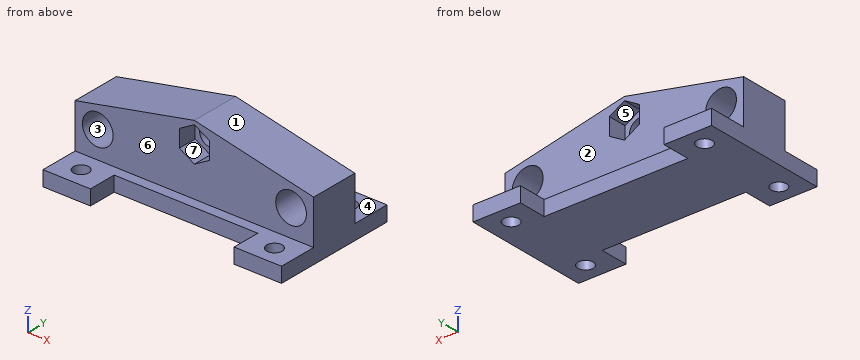
```python
from build123d import *

# Parameters (mm, degrees)
F0_W      = 100.584
F0_H      = 53.34
F1_DEPTH  = 6.35
F2_W      = 100.584
F2_H      = 20.828
F3_DEPTH  = 29.21
F5_DEPTH  = 8
F7_DEPTH  = 8
F9_D      = 9
F11_D     = 12.954
F13_D     = 6.528
F14_W     = 60.584
F14_H     = 12
F15_DEPTH = 6.35
F16_W     = 60.584
F16_H     = 12
F17_DEPTH = 6.35
F19_DEPTH = 20.828


with BuildPart() as f1:
    # F0 (on Top) → F1 (new body)
    with BuildSketch(Plane.XY):
        with Locations((2.149524, 1.085451)):
            Rectangle(F0_W, F0_H)
    extrude(amount=F1_DEPTH)

    # F2 (on face) → F3 (join)
    with BuildSketch(Plane.XY.offset(6.35)):
        with Locations((2.149524, 1.085451)):
            Rectangle(F2_W, F2_H)
    extrude(amount=F3_DEPTH)

    # F4 (on face) → F5 (cut)
    with BuildSketch(Plane.XZ.offset(9.328549)):
        Polygon((8.489524, 23.020798), (8.489524, 30.341599), (2.149524, 34.002), (-4.190476, 30.341599), (-4.190476, 23.020798), (2.149524, 19.360397), align=None)
    extrude(amount=-F5_DEPTH, mode=Mode.SUBTRACT)

    # F6 (on face) → F7 (cut)
    with BuildSketch(Plane(origin=(0, 11.499451, 0), x_dir=(-1, 0, 0), z_dir=(0, 1, 0))):
        Polygon((4.190476, 23.020798), (4.190476, 30.341599), (-2.149524, 34.002), (-8.489524, 30.341599), (-8.489524, 23.020798), (-2.149524, 19.360397), align=None)
    extrude(amount=-F7_DEPTH, mode=Mode.SUBTRACT)

    # F9 (through all)
    with Locations(Plane(origin=(0, 11.499451, 0), x_dir=(-1, 0, 0), z_dir=(0, 1, 0))):
        with Locations((-2.149524, 26.681199)):
            Hole(F9_D / 2)

    # F11 (through all)
    with Locations(Plane.XZ.offset(9.328549)):
        with Locations((42.916524, 17.656), (-38.617476, 17.656)):
            Hole(F11_D / 2)

    # F13 (through all)
    with Locations(Plane.XY.offset(6.35)):
        with Locations((-38.617476, -17.710549), (-38.617476, 19.881451), (42.916524, 19.881451), (42.916524, -17.710549)):
            Hole(F13_D / 2)

    # F14 (on face) → F15 (cut, through all)
    with BuildSketch(Plane.XY.offset(6.35)):
        with Locations((2.149524, 21.755451)):
            Rectangle(F14_W, F14_H)
    extrude(amount=-F15_DEPTH, mode=Mode.SUBTRACT)

    # F16 (on face) → F17 (cut, through all)
    with BuildSketch(Plane.XY.offset(6.35)):
        with Locations((2.149524, -19.584549)):
            Rectangle(F16_W, F16_H)
    extrude(amount=-F17_DEPTH, mode=Mode.SUBTRACT)

    # F18 (on face) → F19 (cut, through all)
    with BuildSketch(Plane.XZ.offset(9.328549)):
        Polygon((-48.142476, 25.013294), (2.149524, 35.56), (-48.142476, 35.56), align=None)
        Polygon((52.441524, 35.56), (2.149524, 35.56), (52.441524, 25.013294), align=None)
    extrude(amount=-F19_DEPTH, mode=Mode.SUBTRACT)


solid = f1.part
```
Verification items for the finished model (mm, model axes). Face numbers are marked on the shaded views. A direction names the side the tool comes from. Coordinates: 2 decimals unless noted, no trailing zeros. Order: outer loops, then holes, each group sorted by start corner. A loop starts at its lowest first (then second) coordinate and runs counter-clockwise, first axis right, second up. Notation, with made-up numbers: (-36, 62) -> (-31, 62) arc R14 cw to (-31, 80) -> close; hole circle Ø6 at (0, 76.25). An arc over 180 degrees is marked (long way). Put each result on its own line as item: value. Start each with the question number.
1) Go/stop test with flat-tipped pins: pin 1 (12 mm diameter, centred on x = -25, z = 22, fed in from +Y); pin 2 (5 mm diameter, centred on x = 12, z = 2, fed in from +Y); pin 3 (10.5 mm diameter, centred on x = -38.62, y = -17.71, fed in from +Z). Record where each tip stops, or that it passes through.
2) Tool access check on the marked faces 4, 5, 6 and 7. Record the directions out of +Z, -Z, +X, -X, +Y, -Y that give a thin tool (end or side, any length) a straight path to the whole face; none if there is none.
3) Cross-section at B-B (y = -16.5). Enter the section's corners in (x, z), plus the area to 3 significant figures.
4) Material ranges on L1, parallel to Y at x = -36, z = 5.5; L2, parallel to X at y = 17, z = 4.5; L3, parallel to Y at x = 9.5, z = 4.5, recorded low to high.
5) Cross-section at A-A (z = 4). Enter the section's corners in (x, y), plus the area to 3 significant figures.
6) Cross-section at D-D (y = 1). Enter the section's corners in (x, z).
7) Release check for a two-part mould opening along X. For the marked faces 1, 2 and 3 record: pulls with the +X half, pulls with the -X half, needs draft (parallel to the pull), parting line crosses it, or undercut.
8) Cross-section at C-C (x = 5). Enter the section's corners in (y, z).
Geometry check:
1. pin 1: stops at y = 11.5
1. pin 2: stops at y = 15.76
1. pin 3: stops at z = 6.35
2. face 4: +Z, +X, -X, +Y
2. face 5: +Y
2. face 6: +Z, +X, -X, -Y
2. face 7: -Y
3. outline: (-48.14, 0) -> (-41.65, 0) -> (-41.65, 6.35) -> (-48.14, 6.35) -> close; (-35.59, 0) -> (-28.14, 0) -> (-28.14, 6.35) -> (-35.59, 6.35) -> close; (32.44, 0) -> (39.89, 0) -> (39.89, 6.35) -> (32.44, 6.35) -> close; (45.95, 0) -> (52.44, 0) -> (52.44, 6.35) -> (45.95, 6.35) -> close
3. area: 177 mm^2
4. L1: y = -25.58 to -19.66, -15.76 to 17.93, 21.83 to 27.76
4. L2: x = -48.14 to -40.15, -37.08 to -28.14, 32.44 to 41.38, 44.45 to 52.44
4. L3: y = -13.58 to 15.76
5. outline: (-48.14, -25.58) -> (-28.14, -25.58) -> (-28.14, -13.58) -> (32.44, -13.58) -> (32.44, -25.58) -> (52.44, -25.58) -> (52.44, 27.76) -> (32.44, 27.76) -> (32.44, 15.76) -> (-28.14, 15.76) -> (-28.14, 27.76) -> (-48.14, 27.76) -> close; hole circle Ø6.53 at (-38.62, -17.71); hole circle Ø6.53 at (-38.62, 19.88); hole circle Ø6.53 at (42.92, -17.71); hole circle Ø6.53 at (42.92, 19.88)
5. area: 3,780 mm^2
6. outline: (-48.14, 0) -> (52.44, 0) -> (52.44, 25.01) -> (2.15, 35.56) -> (-48.14, 25.01) -> close; hole circle Ø12.95 at (-38.62, 17.66); hole circle Ø9 at (2.15, 26.68); hole circle Ø12.95 at (42.92, 17.66)
7. face 1: pulls with the +X half
7. face 2: needs draft
7. face 3: undercut
8. outline: (-13.58, 0) -> (15.76, 0) -> (15.76, 6.35) -> (11.5, 6.35) -> (11.5, 21.01) -> (3.5, 21.01) -> (3.5, 23.2) -> (-1.33, 23.2) -> (-1.33, 21.01) -> (-9.33, 21.01) -> (-9.33, 6.35) -> (-13.58, 6.35) -> close; (-9.33, 32.36) -> (-1.33, 32.36) -> (-1.33, 30.16) -> (3.5, 30.16) -> (3.5, 32.36) -> (11.5, 32.36) -> (11.5, 34.96) -> (-9.33, 34.96) -> close
